Here's how the part is built. I have some questions about the finished solid (model axes, mm). A direction names the side the tool comes from. Round coordinates to 2 decimals unless told otherwise and drop trailing zeros. Loops run counter-clockwise (first coordinate to the right, second up) from the corner with the lowest first, then second, coordinate; pieces in that order, holes last. Notation, with made-up numbers: M 1.5,75 L 23.5,75 A20 cw 23.5,86 Z; hole C 4,60.25 d8. An arc over 180 degrees is marked long. Answer as a JSON object with one key per item and string values.
from build123d import *

# Parameters (mm, degrees)
AUFSATZ_LINEAR_AUSTRAGEN1_DEPTH = 3
VERRUNDUNG1_R                   = 25
VERRUNDUNG2_R                   = 3
SKIZZE3_R                       = 8.5
SCHNITT_LINEAR_AUSTRAGEN1_DEPTH = 49.848849018
SCHNITT_LINEAR_AUSTRAGEN4_DEPTH = 4
SKIZZE4_R                       = 1.5
SKIZZE4_R_2                     = 1.7
SCHNITT_LINEAR_AUSTRAGEN2_DEPTH = 49.848849018
SCHNITT_LINEAR_AUSTRAGEN3_DEPTH = 49.848849018


with BuildPart() as part:
    # Skizze2 → Aufsatz-Linear austragen1 (new body)
    with BuildSketch(Plane.XY):
        with BuildLine():
            Line((-21, -19.807611845), (-21, 19.807611845))
            Line((-21, 19.807611845), (-30.482365961, 29.565355279))
            ThreePointArc((-30.482365961, 29.565355279), (-27.606601718, 35.606601718), (-21.565355279, 38.482365961))
            Line((-21.565355279, 38.482365961), (-11.807611845, 29))
            Line((-11.807611845, 29), (11.807611845, 29))
            Line((11.807611845, 29), (21.565355279, 38.482365961))
            ThreePointArc((21.565355279, 38.482365961), (27.606601718, 35.606601718), (30.482365961, 29.565355279))
            Line((30.482365961, 29.565355279), (21, 19.807611845))
            Line((21, 19.807611845), (21, -19.807611845))
            Line((21, -19.807611845), (30.482365961, -29.565355279))
            ThreePointArc((30.482365961, -29.565355279), (27.606601718, -35.606601718), (21.565355279, -38.482365961))
            Line((21.565355279, -38.482365961), (11.807611845, -29))
            Line((11.807611845, -29), (-11.807611845, -29))
            Line((-11.807611845, -29), (-21.565355279, -38.482365961))
            ThreePointArc((-21.565355279, -38.482365961), (-27.606601718, -35.606601718), (-30.482365961, -29.565355279))
            Line((-30.482365961, -29.565355279), (-21, -19.807611845))
        make_face()
    extrude(amount=AUFSATZ_LINEAR_AUSTRAGEN1_DEPTH)

    # Verrundung1
    verrundung1_edges = [part.edges().sort_by_distance(p)[0] for p in [
        (-21, -19.807611845, 1.5),
        (-21, 19.807611845, 1.5),
        (-11.807611845, 29, 1.5),
        (11.807611845, 29, 1.5),
        (21, 19.807611845, 1.5),
        (21, -19.807611845, 1.5),
        (11.807611845, -29, 1.5),
        (-11.807611845, -29, 1.5),
    ]]
    fillet(verrundung1_edges, radius=VERRUNDUNG1_R)

    # Verrundung2
    verrundung2_edges = [part.edges().sort_by_distance(p)[0] for p in [
        (-30.482365961, 29.565355279, 1.5),
        (-21.565355279, 38.482365961, 1.5),
        (21.565355279, 38.482365961, 1.5),
        (30.482365961, 29.565355279, 1.5),
        (30.482365961, -29.565355279, 1.5),
        (21.565355279, -38.482365961, 1.5),
        (-21.565355279, -38.482365961, 1.5),
        (-30.482365961, -29.565355279, 1.5),
    ]]
    fillet(verrundung2_edges, radius=VERRUNDUNG2_R)

    # Skizze3 → Schnitt-Linear austragen1 (cut, through all)
    with BuildSketch(Plane(origin=(0, 0, 0), x_dir=(-1, 0, 0), z_dir=(0, 0, -1))):
        Circle(SKIZZE3_R)
    extrude(amount=-SCHNITT_LINEAR_AUSTRAGEN1_DEPTH, mode=Mode.SUBTRACT)

    # Skizze7 → Schnitt-Linear austragen4 (cut)
    with BuildSketch(Plane.XY.offset(3)):
        with BuildLine():
            Line((-1.5, 8.948929172), (-7, 5.773502692))
            ThreePointArc((-7, 5.773502692), (-8.098076211, 4.675426481), (-8.5, 3.175426481))
            Line((-8.5, 3.175426481), (-8.5, -3.175426481))
            ThreePointArc((-8.5, -3.175426481), (-8.098076211, -4.675426481), (-7, -5.773502692))
            Line((-7, -5.773502692), (-1.5, -8.948929172))
            ThreePointArc((-1.5, -8.948929172), (0, -9.350852961), (1.5, -8.948929172))
            Line((1.5, -8.948929172), (7, -5.773502692))
            ThreePointArc((7, -5.773502692), (8.098076211, -4.675426481), (8.5, -3.175426481))
            Line((8.5, -3.175426481), (8.5, 3.175426481))
            ThreePointArc((8.5, 3.175426481), (8.098076211, 4.675426481), (7, 5.773502692))
            Line((7, 5.773502692), (1.5, 8.948929172))
            ThreePointArc((1.5, 8.948929172), (0, 9.350852961), (-1.5, 8.948929172))
        make_face()
    extrude(amount=-SCHNITT_LINEAR_AUSTRAGEN4_DEPTH, mode=Mode.SUBTRACT)

    # Skizze4 → Schnitt-Linear austragen2 (cut, through all)
    with BuildSketch(Plane(origin=(0, 0, 0), x_dir=(-1, 0, 0), z_dir=(0, 0, -1))):
        with Locations((-23.363961031, 31.363961031)):
            Circle(SKIZZE4_R)
        with Locations((-17, 25)):
            Circle(SKIZZE4_R)
        with Locations((-15.25, 15.25)):
            Circle(SKIZZE4_R_2)
        with Locations((-17, -25)):
            Circle(SKIZZE4_R)
        with Locations((-15.25, -15.25)):
            Circle(SKIZZE4_R_2)
        with Locations((-23.363961031, -31.363961031)):
            Circle(SKIZZE4_R)
        with Locations((23.363961031, -31.363961031)):
            Circle(SKIZZE4_R)
        with Locations((17, -25)):
            Circle(SKIZZE4_R)
        with Locations((15.25, -15.25)):
            Circle(SKIZZE4_R_2)
        with Locations((23.363961031, 31.363961031)):
            Circle(SKIZZE4_R)
        with Locations((17, 25)):
            Circle(SKIZZE4_R)
        with Locations((15.25, 15.25)):
            Circle(SKIZZE4_R_2)
    extrude(amount=-SCHNITT_LINEAR_AUSTRAGEN2_DEPTH, mode=Mode.SUBTRACT)

    # Skizze5 → Schnitt-Linear austragen3 (cut, through all)
    with BuildSketch(Plane.XY.offset(3)):
        with BuildLine():
            Line((18, 9), (18, -9))
            ThreePointArc((18, -9), (17, -10), (16, -9))
            Line((16, -9), (16, 9))
            ThreePointArc((16, 9), (17, 10), (18, 9))
        make_face()
        with BuildLine():
            Line((-16, 9), (-16, -9))
            ThreePointArc((-16, -9), (-17, -10), (-18, -9))
            Line((-18, -9), (-18, 9))
            ThreePointArc((-18, 9), (-17, 10), (-16, 9))
        make_face()
    extrude(amount=-SCHNITT_LINEAR_AUSTRAGEN3_DEPTH, mode=Mode.SUBTRACT)


solid = part.part
Item 1: I want a section at A-A on y = 1. List the corners of the cut face in (x, z) for me.
Solution:
{"outline": "M -21,0 L -18,0 L -18,3 L -21,3 Z; M -16,0 L -8.5,0 L -8.5,3 L -16,3 Z; M 8.5,0 L 16,0 L 16,3 L 8.5,3 Z; M 18,0 L 21,0 L 21,3 L 18,3 Z"}
Item 2: We'd pull the mould along Y, two halves only. Please class faces 1 (the face through (-6, 9, 3)), 2 (the face through (-16.82, -15.9, 1.48)), 3 (the face through (-21.84, -38.16, 1.52)), 4 (the face through (10.938, 30.785, 1.521)): +Y half, -Y half, draft (parallel to the pull), parting line (faces both ways), or undercut.
Solution:
{"face 1": "draft", "face 2": "undercut", "face 3": "-Y half", "face 4": "+Y half"}
Item 3: If I drill on L1, parallel to X at y = 2.5, z = 1.85; L2, parallel to Y at x = -17, z = 2.35; L3, parallel to Y at x = -15.25, z = 1.15, over which ranges is the centre line in solid material (lowest first)? Write a range as from..to.
Solution:
{"L1": "x = -21..-18, -16..-8.5, 8.5..16, 18..21", "L2": "y = -34.26..-26.5, -23.5..-10, 10..23.5, 26.5..34.26", "L3": "y = -33.02..-16.95, -13.55..13.55, 16.95..33.02"}
Item 4: I want a section at D-D on x = 9.5. List the corners of the cut face in (y, z) for me.
Solution:
{"outline": "M -30.26,0 L 30.26,0 L 30.26,3 L -30.26,3 Z"}
Item 5: I want a section at C-C on z = 1.1. Count the separate pieces of the cut face and the enclosed holes in it, plus the area to 3 significant figures.
Solution:
{"separate pieces": "1", "enclosed holes": "15", "area": "2,720 mm2"}
Item 6: For faces 5 (the face through (-0.02, -9.35, 1.52)), 6 (the face through (-22.785, 18.938, 1.521)), 7 (the face through (21, 0, 1)), which set-ups out of +Z, -Z, +X, -X, +Y, -Y let a thin tool reach every point of the face, with its end or its side?
Solution:
{"face 5": "+Z, -Z", "face 6": "+Z, -Z, -X", "face 7": "+Z, -Z, +X"}
Item 7: For P1, Ø1, axis at y = -27.5, z = 2, coming from the -X side; P2, Ø1.5, axis at y = -1.5, z = 2, coming from the -X side; P3, Ø2, axis at x = -15.25, y = -15.25, coming from the +Z side, each with a flat end and sliding along its axis, tell me the tip position at first contact or that it passes through.
Solution:
{"P1": "stops at x = -28.96", "P2": "stops at x = -21", "P3": "passes through"}
Item 8: I want a section at B-B on y = 15.25. List the corners of the cut face in (x, z) for me.
Solution:
{"outline": "M -21.63,0 L -16.95,0 L -16.95,3 L -21.63,3 Z; M -13.55,0 L 13.55,0 L 13.55,3 L -13.55,3 Z; M 16.95,0 L 21.63,0 L 21.63,3 L 16.95,3 Z"}
